Input: part model. Units: mm. Frame: model coordinates. Coordinates: 2 decimals unless noted, no trailing zeros. Loops run counter-clockwise (first coordinate to the right, second up) from the corner with the lowest first, then second, coordinate; pieces in that order, holes last. Notation, with made-up numbers: (33.25, 51) - (52.25, 51) arc R27 ccw to (52.25, 86) - close; hole circle Ø2 at (-15.75, 14). An arc over 180 degrees is marked (long way). Write item = value, one per line. Start each with the question number.
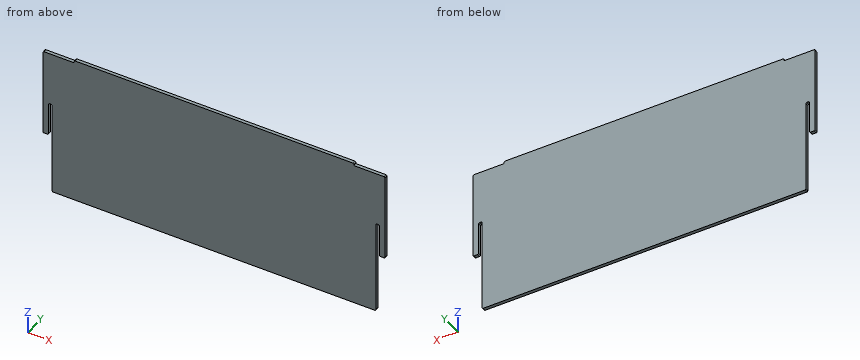
from build123d import *

# Parameters (mm, degrees)
BOSS_EXTRUDE1_DEPTH = 3.175
BOSS_EXTRUDE2_DEPTH = 3.175
FILLET1_R           = 1


with BuildPart() as part:
    # Sketch1 → Boss-Extrude1 (new body)
    with BuildSketch(Plane(origin=(0, 0, 0), x_dir=(1, 0, 0), z_dir=(0, 1, 0))):
        Polygon((292.07333, 0), (313.36742, 0), (313.36742, 143.6878), (0, 143.6878), (0, 0), (21.29409, 0), (21.29409, -2.286), (292.07333, -2.286), align=None)
    extrude(amount=BOSS_EXTRUDE1_DEPTH)

    # Sketch2 → Boss-Extrude2 (add, through all)
    with BuildSketch(Plane(origin=(0, 3.175, 0), x_dir=(1, 0, 0), z_dir=(0, 1, 0))):
        Polygon((0, 0), (-8.926719258, 0), (-8.926719258, 85.152975238), (-3.556, 85.152975238), (-3.556, 52.479835837), (0, 52.479835837), align=None)
        Polygon((313.36742, 52.479835837), (316.92342, 52.479835837), (316.92342, 85.152975238), (322.294139258, 85.152975238), (322.294139258, 0), (313.36742, 0), align=None)
    extrude(amount=-BOSS_EXTRUDE2_DEPTH)

    # Fillet1
    fillet1_edges = [part.edges().sort_by_distance(p)[0] for p in [
        (0, 1.5875, -143.6878),
        (313.36742, 1.5875, -143.6878),
        (292.07333, 1.5875, 2.286),
        (21.29409, 1.5875, 2.286),
        (0, 1.5875, -52.479835837),
        (-8.926719258, 1.5875, 0),
        (-8.926719258, 1.5875, -85.152975238),
        (-3.556, 1.5875, -85.152975238),
        (-3.556, 1.5875, -52.479835837),
        (313.36742, 1.5875, -52.479835837),
        (316.92342, 1.5875, -52.479835837),
        (316.92342, 1.5875, -85.152975238),
        (322.294139258, 1.5875, -85.152975238),
        (322.294139258, 1.5875, 0),
    ]]
    fillet(fillet1_edges, radius=FILLET1_R)


solid = part.part
Item 1: Cut plane C-C on x = 300.5. Return loops of the section in (y, z) (3 decimals), plus the area to 3 significant figures.
Item 2: Ray query, line 1 (X direction, y = 1.6, z = -60); line 2 (Z direction, x = 293, y = 0.65); line 3 (X direction, y = 2.75, z = -135.5). Return the intervals inside material, ascending.
Item 3: Cut plane D-D on z = -114. Return loops of the section in (x, y) (3 decimals).
Item 4: Cut plane A-A on z = -61. Return loops of the section in (x, y) (3 decimals), plus the area to 3 significant figures.
Item 5: Pin query (flat end, axial travel): pin 1 (1.2 mm diameter, centred on x = 315.5, y = 1.5, fed in from -Z); pin 2 (1.6 mm diameter, centred on y = 1.5, z = -104.5, fed in from -X); pin 3 (6 mm diameter, centred on x = 97.5, z = -12.5, fed in from -Y); pin 4 (1 mm diameter, centred on x = 310.5, y = 1.5, fed in from +Z). Return the tip coordinate at first contact, or that it passes through.
Recorded:
q1.outline = (0, -143.688) - (3.175, -143.688) - (3.175, 0) - (0, 0) - close
q1.area = 456 mm²
q2.line_1 = -8.93 to -3.56, 0 to 313.37, 316.92 to 322.29
q2.line_2 = -143.69 to 0
q2.line_3 = 0 to 313.37
q3.outline = (0, 0) - (313.367, 0) - (313.367, 3.175) - (0, 3.175) - close
q4.outline = (-8.927, 0) - (-3.556, 0) - (-3.556, 3.175) - (-8.927, 3.175) - close; (0, 0) - (313.367, 0) - (313.367, 3.175) - (0, 3.175) - close; (316.923, 0) - (322.294, 0) - (322.294, 3.175) - (316.923, 3.175) - close
q4.area = 1,030 mm²
q5.pin_1 = -52.5
q5.pin_2 = 0
q5.pin_3 = 0
q5.pin_4 = 0
